Geometry: see drawing. Coordinates: mm, zero at the bounding-box minimum. A direction names the side the tool comes from. Coordinates: 2 decimals unless noted, no trailing zeros. Write each loop counter-clockwise with the first axis right and the second up, starting at its lowest first coordinate (ties: lowest second). Pieces come first, ordered by that corner, then holes. Notation, with made-up numbers: (5.25, -28.75) - (28.25, -28.75) arc R29 ccw to (28.25, 7.25) - close; hole circle Ø4 at (5, -19). An arc over 180 degrees is marked (long way). Use a Markdown table: item, result. Add a question column.
Q1. Mould query, pull axis Y, two halves, no side actions, for the marked faces 4, 5, 6 and 7. Classes: released by +Y, released by -Y, zero draft, split by the parting line, or undercut.
Q2. Section query D-D (x = 59). Return the cut outline in (y, z).
Q3. Pin query (flat end, axial travel): P1, Ø3, axis at y = 41, z = 118.5, coming from the +X side; P2, Ø8, axis at x = 4, z = 81.5, coming from the +Y side; P3, Ø8, axis at y = 22.5, z = 16, coming from the +X side. Return the tip coordinate at first contact, or that it passes through.
Q4. Set-up query: the marked faces 1, 2 and 3. Return all of +Z, -Z, +X, -X, +Y, -Y with unobstructed straight access to the full face (end or side cutting, diameter ignored); none if empty.
Q5. Section query A-A (y = 144.5). Return the cut outline in (x, z), then the cut area to 3 significant figures.
Q6. Material intervals for probe 1 along Y at (x, z) = (65.25, 70); probe 2 along X at (y, z) = (111.5, 109); probe 3 along Z at (x, y) = (64, 13), sorted ascending. Write a range as from..to.
Q7. Section query C-C (y = 35). Return the cut outline in (x, z).
Q8. Section query B-B (x = 40). Return the cut outline in (y, z), then the cut area to 3 significant figures.
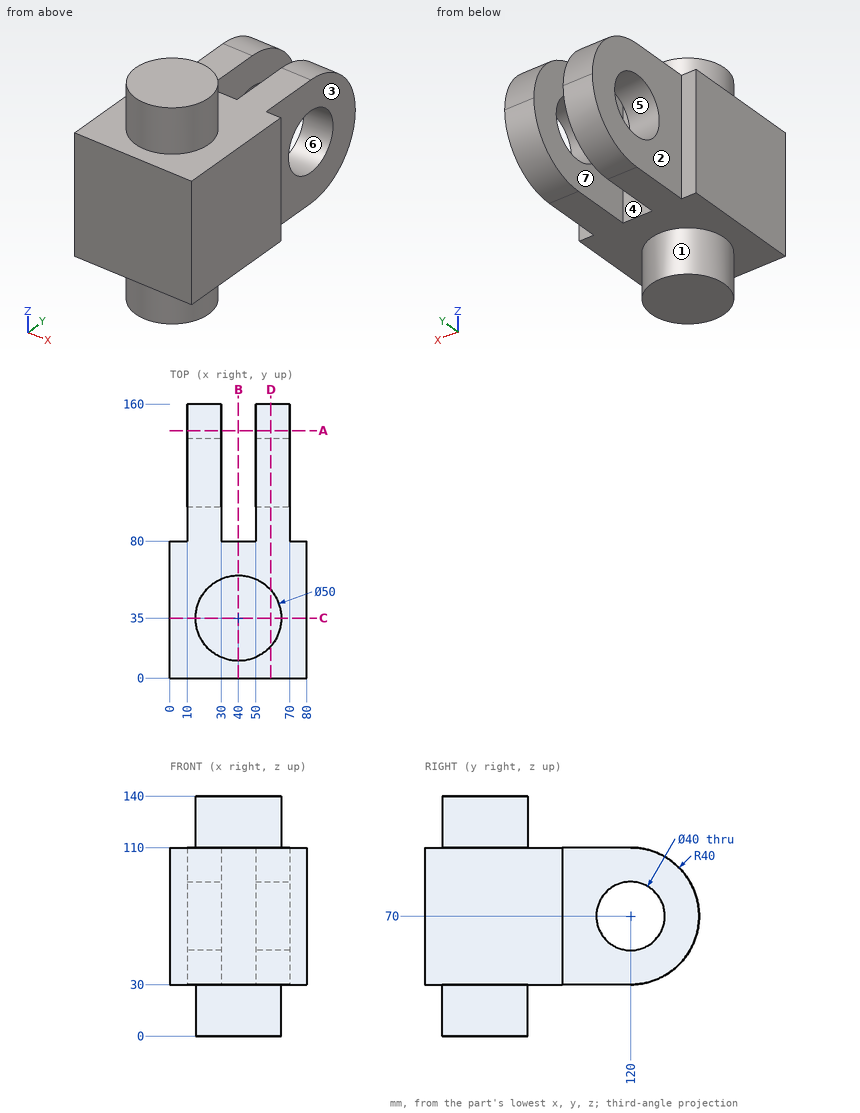
Values follow:
| question | item | result |
|---|---|---|
| 1 | face 4 | released by +Y |
| 1 | face 5 | undercut |
| 1 | face 6 | undercut |
| 1 | face 7 | zero draft |
| 2 | outline | (0, 30) - (18.75, 30) - (18.75, 0) - (51.25, 0) - (51.25, 30) - (120, 30) arc R40 ccw to (120, 110) - (51.25, 110) - (51.25, 140) - (18.75, 140) - (18.75, 110) - (0, 110) - close; hole circle Ø40 at (120, 70) |
| 3 | P1 | x = 64.59 |
| 3 | P2 | y = 80 |
| 3 | P3 | x = 63.51 |
| 4 | face 1 | -Z |
| 4 | face 2 | +Z, -Z, -X, +Y |
| 4 | face 3 | +Z, -Z, +X, +Y |
| 5 | outline | (10, 38.38) - (30, 38.38) - (30, 101.62) - (10, 101.62) - close; (50, 38.38) - (70, 38.38) - (70, 101.62) - (50, 101.62) - close |
| 5 | area | 2,530 mm2 |
| 6 | probe 1 | 0..100, 140..160 |
| 6 | probe 2 | 10..30, 50..70 |
| 6 | probe 3 | 30..110 |
| 7 | outline | (0, 30) - (15, 30) - (15, 0) - (65, 0) - (65, 30) - (80, 30) - (80, 110) - (65, 110) - (65, 140) - (15, 140) - (15, 110) - (0, 110) - close |
| 8 | outline | (0, 30) - (10, 30) - (10, 0) - (60, 0) - (60, 30) - (80, 30) - (80, 110) - (60, 110) - (60, 140) - (10, 140) - (10, 110) - (0, 110) - close |
| 8 | area | 9,400 mm2 |
